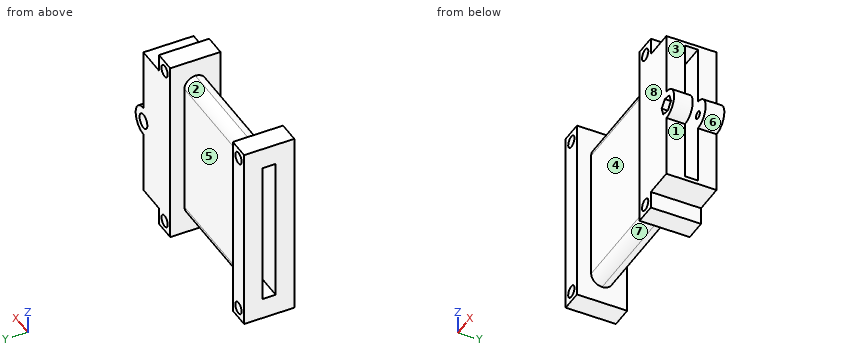
from build123d import *

# Parameters (mm, degrees)
SKETCH1_W           = 42
SKETCH1_H           = 5.9
SKETCH1_W_2         = 39.9
SKETCH1_H_2         = 3.5
BOSS_EXTRUDE1_DEPTH = 32.25
FILLET2_R           = 3
SKETCH2_W           = 51.5
SKETCH2_H           = 13.6
SKETCH2_W_2         = 39.9
SKETCH2_H_2         = 3.5
BOSS_EXTRUDE2_DEPTH = 5.8
SKETCH3_W           = 51.5
SKETCH3_H           = 13.6
SKETCH3_W_2         = 39.9
SKETCH3_H_2         = 3.5
BOSS_EXTRUDE3_DEPTH = 5.8
SKETCH4_R           = 1.6
CUT_EXTRUDE1_DEPTH  = 62.792596644
BOSS_EXTRUDE4_DEPTH = 13.6
CUT_EXTRUDE4_DEPTH  = 4
SKETCH15_W          = 39.9
SKETCH15_H          = 3.5
CUT_EXTRUDE5_DEPTH  = 74.483654645


with BuildPart() as part:
    # Sketch1 → Boss-Extrude1 (new body)
    with BuildSketch(Plane(origin=(0, 0, 0), x_dir=(0, 0, -1), z_dir=(1, 0, 0))):
        with Locations((21, 2.95)):
            Rectangle(SKETCH1_W, SKETCH1_H)
        with Locations((21, 2.95)):
            Rectangle(SKETCH1_W_2, SKETCH1_H_2, mode=Mode.SUBTRACT)
    extrude(amount=BOSS_EXTRUDE1_DEPTH)

    # Fillet2
    # the kernel refuses this fillet: 3 mm, written as the material it takes off along each edge
    with BuildSketch(Plane(origin=(-7.5, 0, -42), x_dir=(0, 0, 1), z_dir=(1, 0, 0)), Plane(origin=(-7.5, 5.9, 0), x_dir=(0, 0, -1), z_dir=(1, 0, 0)), Plane(origin=(-7.5, 5.9, -42), x_dir=(0, -1, 0), z_dir=(1, 0, 0))) as fillet2_piece_1:
        with BuildLine():
            CenterArc((FILLET2_R, -FILLET2_R), FILLET2_R, 90, 90)
            Line((0, -FILLET2_R), (0, 0))
            Line((0, 0), (FILLET2_R, 0))
        make_face()
    extrude(amount=47.25, mode=Mode.SUBTRACT)
    with BuildSketch(Plane(origin=(-7.5, 0, 0), x_dir=(0, 0, -1), z_dir=(1, 0, 0))) as fillet2_piece_2:
        with BuildLine():
            CenterArc((FILLET2_R, FILLET2_R), FILLET2_R, 180, 90)
            Line((0, FILLET2_R), (0, 0))
            Line((0, 0), (FILLET2_R, 0))
        make_face()
    extrude(amount=47.25, mode=Mode.SUBTRACT)

    # Sketch2 → Boss-Extrude2 (add)
    with BuildSketch(Plane(origin=(32.25, 0, 0), x_dir=(0, 0, -1), z_dir=(1, 0, 0))):
        with Locations((21, 2.95)):
            Rectangle(SKETCH2_W, SKETCH2_H)
        with Locations((21, 2.95)):
            Rectangle(SKETCH2_W_2, SKETCH2_H_2, mode=Mode.SUBTRACT)
    extrude(amount=BOSS_EXTRUDE2_DEPTH)

    # Sketch3 → Boss-Extrude3 (add)
    with BuildSketch(Plane.ZY):
        with Locations((-21, 2.95)):
            Rectangle(SKETCH3_W, SKETCH3_H)
        with Locations((-21, 2.95)):
            Rectangle(SKETCH3_W_2, SKETCH3_H_2, mode=Mode.SUBTRACT)
    extrude(amount=BOSS_EXTRUDE3_DEPTH)

    # Sketch4 → Cut-Extrude1 (cut, through all)
    with BuildSketch(Plane(origin=(0, 9.75, 0), x_dir=(1, 0, 0), z_dir=(0, 1, 0))):
        with Locations(Location((-2.9, 43.85, 0), (0, 0, 270))):
            Circle(SKETCH4_R)
        with Locations(Location((35.15, 43.85, 0), (0, 0, 270))):
            Circle(SKETCH4_R)
        with Locations(Location((-2.9, -1.85, 0), (0, 0, 270))):
            Circle(SKETCH4_R)
        with Locations(Location((35.15, -1.85, 0), (0, 0, 270))):
            Circle(SKETCH4_R)
    extrude(amount=-CUT_EXTRUDE1_DEPTH, mode=Mode.SUBTRACT)

    # Sketch8 → Boss-Extrude4 (add)
    with BuildSketch(Plane(origin=(0, 9.75, 0), x_dir=(1, 0, 0), z_dir=(0, 1, 0))):
        with BuildLine():
            ThreePointArc((46.05, 17), (50.05, 21), (46.05, 25))
            Line((46.05, 25), (46.05, 41.999583304))
            Line((46.05, 41.999583304), (38.05, 41.999583304))
            Line((38.05, 41.999583304), (38.05, 0.000416696))
            Line((38.05, 0.000416696), (46.05, 0.000416696))
            Line((46.05, 0.000416696), (46.05, 17))
        make_face()
    extrude(amount=-BOSS_EXTRUDE4_DEPTH)

    # Sketch13 → CSK for M2 Flat Head Machine Screw1 (revolve, cut)
    with BuildSketch(Plane(origin=(46.05, 9.75, -21), x_dir=(0, 0, 1), z_dir=(1, 0, 0))):
        Polygon((0, 0), (0, 13.6), (1, 13.6), (1, 3.75), (2, 2.75), (2, 0), align=None)
    revolve(axis=Axis((46.05, 16.1, -21), (0, -1, 0)), mode=Mode.SUBTRACT)

    # Sketch14 → Cut-Extrude4 (cut)
    with BuildSketch(Plane.XZ.offset(3.85)):
        Polygon((43.671623782, -20.5274256), (44.451550455, -22.823447025), (46.829926673, -23.296021425), (48.428376218, -21.4725744), (47.648449545, -19.176552975), (45.270073327, -18.703978575), align=None)
    extrude(amount=-CUT_EXTRUDE4_DEPTH, mode=Mode.SUBTRACT)

    # Sketch15 → Cut-Extrude5 (cut, through all)
    with BuildSketch(Plane.ZY.offset(5.8)):
        with Locations((-21, 2.95)):
            Rectangle(SKETCH15_W, SKETCH15_H)
    extrude(amount=-CUT_EXTRUDE5_DEPTH, mode=Mode.SUBTRACT)


solid = part.part
The model under review builds one solid part; all positions refer to its coordinate system, in mm. Face numbers are marked on the shaded views. A direction names the side the tool comes from. Give positions to 0.01 mm unless a question says otherwise; leave off trailing zeros. Order: outer loops, then holes, each group sorted by start corner. A loop starts at its lowest first (then second) coordinate and runs counter-clockwise, first axis right, second up. Notation, with made-up numbers: M 61,36 L 78,36 A19 ccw 78,63 Z; hole C 38.5,47.5 d7. An arc over 180 degrees is marked long. One line per question, with ' | ' between items. Start each with the question number.
1) Clearance check with flat-ended pins moving along their axes: P1, Ø3, axis at x = 28.5, z = -11, coming from the +Y side; P2, Ø1, axis at x = 14.5, y = 3.5, coming from the +Z side; P3, Ø4, axis at x = 43, y = 1.5, coming from the -Z side; P4, Ø4, axis at y = 1.5, z = -9, coming from the -X side. State where each tip first meets the part, or that it passes through.
2) For the marked faces 1, 2, 3, 4 and 5, list the 3-axis set-ups (+Z, -Z, +X, -X, +Y, -Y) from which the entire face can be reached by the end or side of a thin tool; tool diameter is ignored.
3) Consider section C-C, the plane z = -43.85. Give the boundary of the cut face in (x, y), then the cut area to 3 significant figures.
4) Wall thickness on L1, parallel to X at y = 0.5, z = -43.85; L2, parallel to Y at x = 27, z = -3.5; L3, parallel to Y at x = -1.5, z = -4.5: over which ranges is each line inside the solid? List them lowest first. Write a range as from..to.
5) Consider section A-A, the plane y = 8.25. Give the boundary of the cut face in (x, z).
6) Consider section D-D, the plane x = 17. Give the boundary of the cut face in (y, z), then the cut area to 3 significant figures.
7) Consider section B-B, the plane x = -2.9. Give the boundary of the cut face in (y, z).
8) Mouldability with a two-part tool opening along X and no side actions: class the marked faces 6, 7 and 8 as pulls with the +X half, pulls with the -X half, needs draft (parallel to the pull), parting line crosses it, or undercut.
Found:
1) P1: stops at y = 5.9 | P2: stops at z = 0 | P3: stops at z = -42 | P4: stops at x = -5.8
2) face 1: -Z, +X, +Y, -Y | face 2: +Z, +Y | face 3: +Z, +X, +Y, -Y | face 4: +Z, -Z, -Y | face 5: +Z, -Z, +Y
3) outline: M -5.8,-3.85 L -4.5,-3.85 L -4.5,9.75 L -5.8,9.75 Z; M -1.3,-3.85 L 0,-3.85 L 0,9.75 L -1.3,9.75 Z; M 32.25,-3.85 L 33.55,-3.85 L 33.55,9.75 L 32.25,9.75 Z; M 36.75,-3.85 L 38.05,-3.85 L 38.05,9.75 L 36.75,9.75 Z | area: 70.7 mm²
4) L1: x = -5.8..-4.5, -1.3..0, 32.25..33.55, 36.75..38.05 | L2: y = 0..1.2, 4.7..5.9 | L3: y = -3.85..1.2, 4.7..9.75
5) outline: M -5.8,-46.75 L 0,-46.75 L 0,4.75 L -5.8,4.75 Z; M 32.25,-46.75 L 38.05,-46.75 L 38.05,-42 L 46.05,-42 L 46.05,-25 A4 ccw 46.05,-17 L 46.05,0 L 38.05,0 L 38.05,4.75 L 32.25,4.75 Z; hole C -2.9,-43.85 d3.2; hole C -2.9,1.85 d3.2; hole C 35.15,-43.85 d3.2; hole C 35.15,1.85 d3.2; hole C 46.05,-21 d4
6) outline: M 0,-39 A3 ccw 2.95,-42 A3 ccw 5.9,-39 L 5.9,-3 A3 ccw 2.95,0 A3 ccw 0,-3 Z; hole M 1.2,-40.95 L 4.7,-40.95 L 4.7,-1.05 L 1.2,-1.05 Z | area: 100 mm²
7) outline: M -3.85,-46.75 L 9.75,-46.75 L 9.75,-45.45 L -3.85,-45.45 Z; M -3.85,-42.25 L 9.75,-42.25 L 9.75,0.25 L -3.85,0.25 Z; M -3.85,3.45 L 9.75,3.45 L 9.75,4.75 L -3.85,4.75 Z; hole M 1.2,-40.95 L 4.7,-40.95 L 4.7,-1.05 L 1.2,-1.05 Z
8) face 6: pulls with the +X half | face 7: undercut | face 8: needs draft
